Read the model definition and answer for the solid it produces. Units are mm, in the model's axes. A direction names the side the tool comes from. Coordinates: 2 decimals unless noted, no trailing zeros. Order: outer loops, then holes, each group sorted by start corner. A loop starts at its lowest first (then second) coordinate and runs counter-clockwise, first axis right, second up. Notation, with made-up numbers: M 49.25,73.5 L 79.25,73.5 A10 cw 79.25,87.5 Z; hole C 73,22 d7. An arc over 180 degrees is marked long. One line per question, with ' | ' between items. Start each with the question number.
1) Find section A-A, the plane x = 0. Write down the section's boundary in (y, z).
2) Consider probe 1 along Z at (x, y) = (6.75, 7); probe 2 along Y at (x, z) = (11, -3.4); probe 3 along Y at (x, z) = (4, -3.9). Determine where each line is inside the solid, lowest interval first.
3) Find section C-C, the plane x = -10.25. Write down the section's boundary in (y, z).
4) Given P1, Ø5, axis at x = 2.5, y = -0.5, coming from the -Z side; P2, Ø1, axis at x = -7, z = -2.5, coming from the +Y side; P3, Ø5.5, axis at x = -11, y = 0, coming from the +Z side; P4, Ø2.5, axis at x = 11, y = 0, coming from the +Z side, each flat-ended and moving along its own axis, determine where each tip first touches the part or whether it passes through.
5) The mould has two halves that part along Y. Classify faces 1 (the face through (0.51, -12.62, -3.44)), 2 (the face through (-8.06, -12.65, -3.46)), 3 (the face through (6, 6, -2.699)): +Y half, -Y half, draft (parallel to the pull), parting line (faces both ways), or undercut.
6) A tool of negligible diameter and unlimited length cuts with its end or side. For faces 4 (the face through (-12.62, -0.51, -3.44)), 5 (the face through (1.73, 7.81, -1.22)), 6 (the face through (1.42, 3.92, -1.699)), from which of +Z, -Z, +X, -X, +Y, -Y can it reach the whole face along a straight path? Write none if from no direction.
7) Find section D-D, the plane y = 11. Write down the section's boundary in (x, z).
from build123d import *

# Parameters (mm, degrees)
M3_CLEARANCE_HOLE1_D = 3.4
CIRPATTERN1_COUNT    = 4


with BuildPart() as part:
    # Sketch1 → Revolve1 (revolve)
    with BuildSketch(Plane(origin=(0, 0, 0), x_dir=(1, 0, 0), z_dir=(0, 1, 0)), mode=Mode.PRIVATE) as revolve1_sk:
        Polygon((4, 1.698663418), (4, -0.301336582), (8, -0.301336582), (8, 2.698663418), (15, 2.698663418), (15, 4.198663418), (6, 4.198663418), (6, 1.698663418), align=None)
    revolve(revolve1_sk.sketch.rotate(Axis((0, 0, -9.651281217), (0, 0, 1)), 180), axis=Axis((0, 0, -9.651281217), (0, 0, 1)))

    # M3 Clearance Hole1 (through all)
    with Locations(Plane(origin=(0, 0, -4.198663418), x_dir=(-1, 0, 0), z_dir=(0, 0, -1))):
        with Locations((-11, 0)):
            m3_clearance_hole1 = Hole(M3_CLEARANCE_HOLE1_D / 2)

    # CirPattern1: M3 Clearance Hole1 ×4 about axis
    cirpattern1_axis = Axis((0, 0, 0), (0, 0, 1))
    for i in range(1, CIRPATTERN1_COUNT):
        add(m3_clearance_hole1.rotate(cirpattern1_axis, i * 360 / CIRPATTERN1_COUNT), mode=Mode.SUBTRACT)


solid = part.part
Report:
1) outline: M -15,-4.2 L -12.7,-4.2 L -12.7,-2.7 L -15,-2.7 Z; M -9.3,-4.2 L -6,-4.2 L -6,-1.7 L -4,-1.7 L -4,0.3 L -8,0.3 L -8,-2.7 L -9.3,-2.7 Z; M 4,-1.7 L 6,-1.7 L 6,-4.2 L 9.3,-4.2 L 9.3,-2.7 L 8,-2.7 L 8,0.3 L 4,0.3 Z; M 12.7,-4.2 L 15,-4.2 L 15,-2.7 L 12.7,-2.7 Z
2) probe 1: z = -4.2 to -2.7 | probe 2: y = -10.2 to -1.7, 1.7 to 10.2 | probe 3: y = -14.46 to -4.47, 4.47 to 14.46
3) outline: M -10.95,-4.2 L -1.53,-4.2 L -1.53,-2.7 L -10.95,-2.7 Z; M 1.53,-4.2 L 10.95,-4.2 L 10.95,-2.7 L 1.53,-2.7 Z
4) P1: stops at z = -1.7 | P2: stops at y = 13.5 | P3: stops at z = -2.7 | P4: passes through
5) face 1: undercut | face 2: parting line | face 3: draft
6) face 4: +Z, -Z | face 5: +Z | face 6: -Z
7) outline: M -10.2,-4.2 L -1.7,-4.2 L -1.7,-2.7 L -10.2,-2.7 Z; M 1.7,-4.2 L 10.2,-4.2 L 10.2,-2.7 L 1.7,-2.7 Z
